Geometry: final body of the model. Coordinates: model frame, mm. A direction names the side the tool comes from. Coordinates: 2 decimals unless noted, no trailing zeros. Write each loop counter-clockwise with the first axis right and the second up, starting at its lowest first coordinate (ties: lowest second). Pieces come first, ordered by that corner, then holes. Notation, with made-up numbers: (30.25, -34.5) -> (54.25, -34.5) arc R33 ccw to (54.25, 1.5) -> close; hole circle Ø10 at (15.25, 64). An arc over 180 degrees is marked (long way). One line per item, written item: value.
```python
from build123d import *

# Parameters (mm, degrees)
SKETCH_1_R          = 1.55
EXTRUDE_4_DEPTH     = 3
EXTRUDE_5_DEPTH     = 33
SKETCH_3_W          = 7
SKETCH_3_H          = 10
CUT_EXTRUDE_1_DEPTH = 6


with BuildPart() as part:
    # Sketch 1 → Extrude 4 (new body)
    with BuildSketch(Plane.XY):
        Polygon((10, -2.75), (10, 0), (50, 0), (90, 0), (90, -2.75), (100, -2.75), (100, 0), (102.75, 0), (102.75, 10), (100, 10), (100, 90), (102.75, 90), (102.75, 100), (100, 100), (100, 102.75), (90, 102.75), (90, 100), (50, 100), (10, 100), (10, 102.75), (0, 102.75), (0, 100), (-2.75, 100), (-2.75, 90), (0, 90), (0, 10), (-2.75, 10), (-2.75, 0), (0, 0), (0, -2.75), align=None)
        with Locations((5, 5)):
            Circle(SKETCH_1_R, mode=Mode.SUBTRACT)
        with Locations((40, 12)):
            Circle(SKETCH_1_R, mode=Mode.SUBTRACT)
        with Locations((12, 40)):
            Circle(SKETCH_1_R, mode=Mode.SUBTRACT)
        with Locations((60, 12)):
            Circle(SKETCH_1_R, mode=Mode.SUBTRACT)
        with Locations((95, 5)):
            Circle(SKETCH_1_R, mode=Mode.SUBTRACT)
        with Locations((88, 40)):
            Circle(SKETCH_1_R, mode=Mode.SUBTRACT)
        with Locations((12, 60)):
            Circle(SKETCH_1_R, mode=Mode.SUBTRACT)
        with Locations((45, 50)):
            Circle(SKETCH_1_R, mode=Mode.SUBTRACT)
        with Locations((5, 95)):
            Circle(SKETCH_1_R, mode=Mode.SUBTRACT)
        with Locations((40, 88)):
            Circle(SKETCH_1_R, mode=Mode.SUBTRACT)
        with Locations((60, 88)):
            Circle(SKETCH_1_R, mode=Mode.SUBTRACT)
        with Locations((55, 50)):
            Circle(SKETCH_1_R, mode=Mode.SUBTRACT)
        with Locations((88, 60)):
            Circle(SKETCH_1_R, mode=Mode.SUBTRACT)
        with Locations((95, 95)):
            Circle(SKETCH_1_R, mode=Mode.SUBTRACT)
    extrude(amount=EXTRUDE_4_DEPTH)

    # Sketch 1_8 → Extrude 5 (add)
    with BuildSketch(Plane.XY):
        Polygon((10, -2.75), (0, -2.75), (0, -6), (100, -6), (100, -2.75), (90, -2.75), align=None)
        with BuildLine():
            Line((100, -2.75), (100, -6))
            ThreePointArc((100, -6), (104.242640687, -4.242640687), (106, 0))
            Line((106, 0), (102.75, 0))
            Line((102.75, 0), (100, 0))
            Line((100, 0), (100, -2.75))
        make_face()
        Polygon((102.75, 0), (106, 0), (106, 100), (102.75, 100), (102.75, 90), (102.75, 10), align=None)
        with BuildLine():
            Line((102.75, 100), (106, 100))
            ThreePointArc((106, 100), (104.242640687, 104.242640687), (100, 106))
            Line((100, 106), (100, 102.75))
            Line((100, 102.75), (100, 100))
            Line((100, 100), (100.25, 100))
            Line((100.25, 100), (102.75, 100))
        make_face()
        Polygon((100, 106), (0, 106), (0, 102.75), (10, 102.75), (90, 102.75), (100, 102.75), align=None)
        with BuildLine():
            ThreePointArc((0, 106), (-4.242640687, 104.242640687), (-6, 100))
            Line((-6, 100), (-2.75, 100))
            Line((-2.75, 100), (0, 100))
            Line((0, 100), (0, 102.75))
            Line((0, 102.75), (0, 106))
        make_face()
        Polygon((-6, 0), (-2.75, 0), (-2.75, 10), (-2.75, 90), (-2.75, 100), (-6, 100), align=None)
        with BuildLine():
            Line((0, -2.75), (0, 0))
            Line((0, 0), (-2.75, 0))
            Line((-2.75, 0), (-6, 0))
            ThreePointArc((-6, 0), (-4.242640687, -4.242640687), (0, -6))
            Line((0, -6), (0, -2.75))
        make_face()
    extrude(amount=EXTRUDE_5_DEPTH)

    # Sketch 3 → Cut-Extrude 1 (cut)
    with BuildSketch(Plane.XZ.offset(-102.75)):
        with Locations((13.5, 13)):
            Rectangle(SKETCH_3_W, SKETCH_3_H)
    extrude(amount=-CUT_EXTRUDE_1_DEPTH, mode=Mode.SUBTRACT)


solid = part.part
```
(1) Pull-direction query (X, two-part tool) for faces 1 (the flat face through (49, 0, 1)), 2 (the cylindrical face through (-4.289, -4.196, 16.269)), 3 (the flat face through (49, -6, 16)); classes: released by +X, released by -X, zero draft, split by the parting line, or undercut.
Responses:
face 1: undercut
face 2: released by -X
face 3: zero draft
(2) First-contact query: pin 1 (4 mm diameter, centred on x = 93, y = 53, fed in from +Z); pin 2 (0.8 mm diameter, centred on y = 101, z = 2, fed in from -X); pin 3 (0.8 mm diameter, centred on x = 102, z = 17, fed in from -Y). Flat tips, straight axial feed; report the tip coordinate or a pass-through.
Responses:
pin 1: stops at z = 3
pin 2: stops at x = -5.97
pin 3: stops at y = -5.78
(3) Section A-A (x = 55). Return the cut outline in (y, z), then the cut area to 3 significant figures.
Responses:
outline: (-6, 0) -> (-2.75, 0) -> (-2.75, 33) -> (-6, 33) -> close; (0, 0) -> (48.45, 0) -> (48.45, 3) -> (0, 3) -> close; (51.55, 0) -> (100, 0) -> (100, 3) -> (51.55, 3) -> close; (102.75, 0) -> (106, 0) -> (106, 33) -> (102.75, 33) -> close
area: 505 mm2
(4) Section B-B (y = 75.5). Return the cut outline in (x, z), then the cut area to 4 significant figures.
Responses:
outline: (-6, 0) -> (-2.75, 0) -> (-2.75, 33) -> (-6, 33) -> close; (0, 0) -> (100, 0) -> (100, 3) -> (0, 3) -> close; (102.75, 0) -> (106, 0) -> (106, 33) -> (102.75, 33) -> close
area: 514.5 mm2
(5) Reachability of faces 4 (the flat face through (101, 100, 18)), 5 (the flat face through (13, 104, 8)), 6 (the flat face through (90, -1, 1)), 7 (the flat face through (50, 104, 33)) from +Z, -Z, +X, -X, +Y, -Y: full face, straight path, thin tool, end or side. Return the list, or none.
Responses:
face 4: +Z
face 5: +Y
face 6: +Z, -Z
face 7: +Z, +X, -X, +Y, -Y
(6) Section D-D (z = 28). Return the cut outline in (x, y).
Responses:
outline: (-6, 0) arc R6 ccw to (0, -6) -> (100, -6) arc R6 ccw to (106, 0) -> (106, 100) arc R6 ccw to (100, 106) -> (0, 106) arc R6 ccw to (-6, 100) -> close; hole (-2.75, 0) -> (0, 0) -> (0, -2.75) -> (100, -2.75) -> (100, 0) -> (102.75, 0) -> (102.75, 100) -> (100, 100) -> (100, 102.75) -> (0, 102.75) -> (0, 100) -> (-2.75, 100) -> close
(7) Line query: line 1 (Y direction, x = 12, z = 2); line 2 (Y direction, x = 45, z = 2.3); line 3 (Y direction, x = 60, z = 2). Output: solid intervals per line, ascending. Write a range as [from, to].
Responses:
line 1: y = [-6, -2.75], [0, 38.45], [41.55, 58.45], [61.55, 100], [102.75, 106]
line 2: y = [-6, -2.75], [0, 48.45], [51.55, 100], [102.75, 106]
line 3: y = [-6, -2.75], [0, 10.45], [13.55, 86.45], [89.55, 100], [102.75, 106]
(8) Section C-C (x = 95). Return the cut outline in (y, z), then the cut area to 3 significant figures.
Responses:
outline: (-6, 0) -> (3.45, 0) -> (3.45, 3) -> (-2.75, 3) -> (-2.75, 33) -> (-6, 33) -> close; (6.55, 0) -> (93.45, 0) -> (93.45, 3) -> (6.55, 3) -> close; (96.55, 0) -> (106, 0) -> (106, 33) -> (102.75, 33) -> (102.75, 3) -> (96.55, 3) -> close
area: 512 mm2
